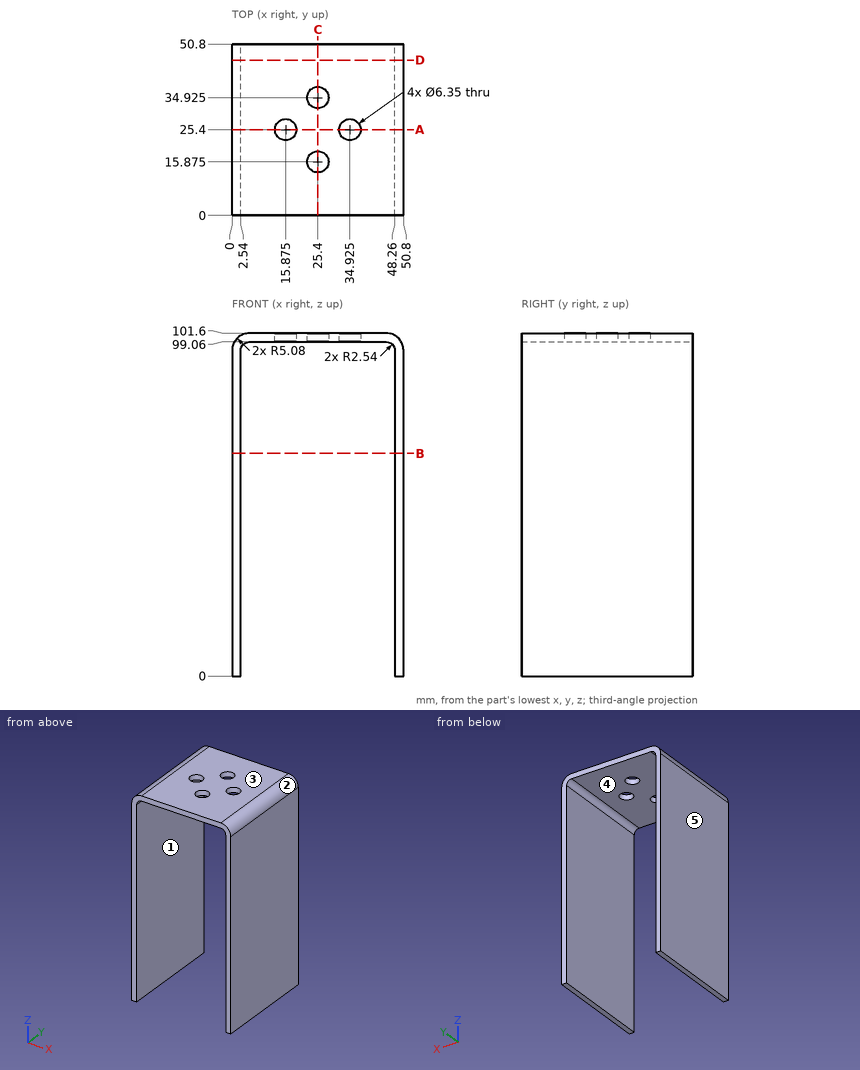
Geometry: see drawing. Coordinates: mm, zero at the bounding-box minimum. A direction names the side the tool comes from. Round coordinates to 2 decimals unless told otherwise and drop trailing zeros. Order: outer loops, then holes, each group sorted by start corner. A loop starts at its lowest first (then second) coordinate and runs counter-clockwise, first axis right, second up. Notation, with made-up numbers: (-35, 57.25) - (-29, 57.25) arc R18 ccw to (-29, 74.25) - close; hole circle Ø6 at (71.25, 36.25). An arc over 180 degrees is marked (long way). Use a Markdown table: item, result. Add a question column.
1. Mould query, pull axis X, two halves, no side actions, for the marked faces 3, 4 and 5. Classes: +X half, -X half, draft (parallel to the pull), parting line (faces both ways), or undercut.
2. Section query A-A (y = 25.4). Return the cut outline in (x, z).
3. Set-up query: the marked faces 1 and 2. Return all of +Z, -Z, +X, -X, +Y, -Y with unobstructed straight access to the full face (end or side cutting, diameter ignored); none if empty.
4. First-contact query: pin 1 (10 mm diameter, centred on x = 15.875, y = 25.4, fed in from -Z); pin 2 (4 mm diameter, centred on x = 34.925, y = 25.4, fed in from -Z). Flat tips, straight axial feed; report the tip coordinate or a pass-through.
5. Section query D-D (y = 46). Return the cut outline in (x, z).
6. Line query: probe 1 along Y at (x, z) = (25.4, 100.65); probe 2 along X at (y, z) = (48, 42.5); probe 3 along Z at (x, y) = (40.5, 18.5). Output: solid intervals per line, ascending.
7. Section query C-C (x = 25.4). Return the cut outline in (y, z).
8. Section query B-B (z = 66). Return the cut outline in (x, y).
Derived:
| question | item | result |
|---|---|---|
| 1 | face 3 | draft |
| 1 | face 4 | undercut |
| 1 | face 5 | -X half |
| 2 | outline | (0, 0) - (2.54, 0) - (2.54, 96.52) arc R2.54 cw to (5.08, 99.06) - (12.7, 99.06) - (12.7, 101.6) - (5.08, 101.6) arc R5.08 ccw to (0, 96.52) - close; (19.05, 99.06) - (31.75, 99.06) - (31.75, 101.6) - (19.05, 101.6) - close; (38.1, 99.06) - (45.72, 99.06) arc R2.54 cw to (48.26, 96.52) - (48.26, 0) - (50.8, 0) - (50.8, 96.52) arc R5.08 ccw to (45.72, 101.6) - (38.1, 101.6) - close |
| 3 | face 1 | -Z, +Y, -Y |
| 3 | face 2 | +Z, +X, +Y, -Y |
| 4 | pin 1 | z = 99.06 |
| 4 | pin 2 | through |
| 5 | outline | (0, 0) - (2.54, 0) - (2.54, 96.52) arc R2.54 cw to (5.08, 99.06) - (45.72, 99.06) arc R2.54 cw to (48.26, 96.52) - (48.26, 0) - (50.8, 0) - (50.8, 96.52) arc R5.08 ccw to (45.72, 101.6) - (5.08, 101.6) arc R5.08 ccw to (0, 96.52) - close |
| 6 | probe 1 | 0 to 12.7, 19.05 to 31.75, 38.1 to 50.8 |
| 6 | probe 2 | 0 to 2.54, 48.26 to 50.8 |
| 6 | probe 3 | 99.06 to 101.6 |
| 7 | outline | (0, 99.06) - (12.7, 99.06) - (12.7, 101.6) - (0, 101.6) - close; (19.05, 99.06) - (31.75, 99.06) - (31.75, 101.6) - (19.05, 101.6) - close; (38.1, 99.06) - (50.8, 99.06) - (50.8, 101.6) - (38.1, 101.6) - close |
| 8 | outline | (0, 0) - (2.54, 0) - (2.54, 50.8) - (0, 50.8) - close; (48.26, 0) - (50.8, 0) - (50.8, 50.8) - (48.26, 50.8) - close |
